Read the model definition and answer for the solid it produces. Units are mm, in the model's axes. A direction names the side the tool comes from. Give positions to 0.01 mm unless a question says otherwise; leave off trailing zeros. Write each loop counter-clockwise with the first axis right and the second up, starting at its lowest first coordinate (ties: lowest second). Pieces come first, ordered by that corner, then holes. Notation, with made-up numbers: M 9.25,53.25 L 61.25,53.25 A17 ccw 61.25,85.25 Z; hole C 4,59.5 d2. An arc over 180 degrees is marked long. Put each result on its own line as item: value.
from build123d import *

# Parameters (mm, degrees)
SKETCH1_R           = 3
BOSS_EXTRUDE1_DEPTH = 32.5
CUT_EXTRUDE1_DEPTH  = 8
CHAMFER1_SIZE       = 0.5


with BuildPart() as part:
    # Sketch1 → Boss-Extrude1 (new body, symmetric)
    with BuildSketch(Plane(origin=(0, 0, 0), x_dir=(0, 0, -1), z_dir=(1, 0, 0))):
        Circle(SKETCH1_R)
    extrude(amount=BOSS_EXTRUDE1_DEPTH, both=True)

    # Sketch2 → Cut-Extrude1 (cut)
    with BuildSketch(Plane(origin=(32.5, 0, 0), x_dir=(0, 0, -1), z_dir=(1, 0, 0))):
        with BuildLine():
            Line((-2.236067977, 2), (2.236067977, 2))
            ThreePointArc((2.236067977, 2), (0, 3), (-2.236067977, 2))
        make_face()
    extrude(amount=-CUT_EXTRUDE1_DEPTH, mode=Mode.SUBTRACT)

    # Chamfer1
    chamfer1_edges = [part.edges().sort_by_distance(p)[0] for p in [
        (-32.5, 0, 3),
        (32.5, -2.802517077, 1.070466269),
        (32.5, 2, 0),
    ]]
    chamfer(chamfer1_edges, length=CHAMFER1_SIZE)


solid = part.part
(1) Which of the six approach directions +Z, -Z, +X, -X, +Y, -Y give full straight-line access (tool end or side, diameter ignored) to faces 1 (the face through (24.5, 2.4, 0)), 2 (the face through (32.365, -2.634, 0.085))?
Result:
face 1: +Z, -Z, +X, +Y
face 2: +X
(2) Section A-A on z = 0 is taken. Determine the outline of the cut face in (x, y).
Result:
outline: M -32.5,-2.5 L -32,-3 L 32,-3 L 32.5,-2.5 L 32.5,1.5 L 32,2 L 24.5,2 L 24.5,3 L -32,3 L -32.5,2.5 Z
(3) Given pin 1 Ø1 at (x, y) = (-21.5, -1.5) entering from +Z; pin 2 Ø2 at (x, z) = (27, 0) entering from +Y; pin 3 Ø1 at (x, y) = (-4, -2) entering from -Z, each flat-ended and moving along its own axis, determine where each tip first touches the part or whether it passes through.
Result:
pin 1: stops at z = 2.83
pin 2: stops at y = 2
pin 3: stops at z = -2.6
(4) Section B-B on x = -12.5 is taken. Determine the outline of the cut face in (y, z).
Result:
outline: C 0,0 d6
(5) Straight lines are drawn through the part: line 1 along X through (y, z) = (2.05, -0.2); line 2 along Z through (x, y) = (-11, 1.65); line 3 along X through (y, z) = (1.8, 0.1). For each, find the intervals that lie inside material, in ascending order. Write a range as from..to.
Result:
line 1: x = -32.5..24.5
line 2: z = -2.51..2.51
line 3: x = -32.5..32.2
